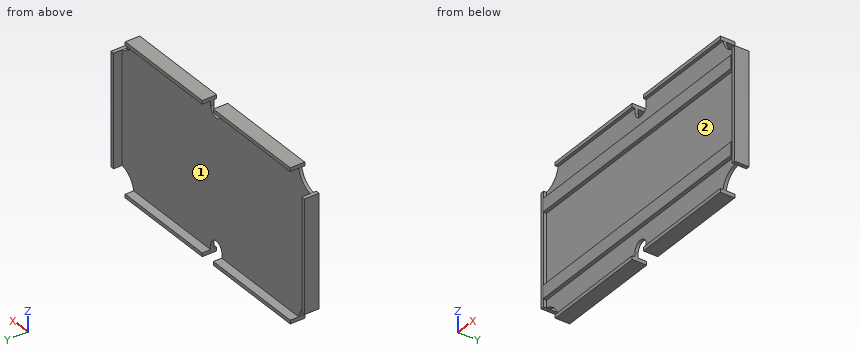
```python
from build123d import *

# Parameters (mm, degrees)
CROQUIS1_W              = 92.4
CROQUIS1_H              = 52.4
SALIENTE_EXTRUIR1_DEPTH = 5
CROQUIS2_W              = 89.9
CROQUIS2_H              = 49.9
CORTAR_EXTRUIR1_DEPTH   = 2.93
CORTAR_EXTRUIR2_START   = -2.07
CORTAR_EXTRUIR2_DEPTH   = 5
CORTAR_EXTRUIR3_START   = -2.07
CORTAR_EXTRUIR3_DEPTH   = 5
SIMETR_A2_START         = -2.07
SIMETR_A2_COPY_1_DEPTH  = 5
CORTAR_EXTRUIR5_DEPTH   = 1
CROQUIS7_W              = 89.9
CROQUIS7_H              = 4.51
SALIENTE_EXTRUIR2_DEPTH = 1.24


with BuildPart() as part:
    # Croquis1 → Saliente-Extruir1 (new body)
    with BuildSketch(Plane(origin=(0, 0, 0), x_dir=(1, 0, 0), z_dir=(0, 1, 0))):
        Rectangle(CROQUIS1_W, CROQUIS1_H)
    extrude(amount=SALIENTE_EXTRUIR1_DEPTH)

    # Croquis2 → Cortar-Extruir1 (cut)
    with BuildSketch(Plane(origin=(0, 5, 0), x_dir=(1, 0, 0), z_dir=(0, 1, 0))):
        Rectangle(CROQUIS2_W, CROQUIS2_H)
    extrude(amount=-CORTAR_EXTRUIR1_DEPTH, mode=Mode.SUBTRACT)

    # Croquis3 → Cortar-Extruir2 (cut)
    with BuildSketch(Plane(origin=(0, 2.07, 0), x_dir=(1, 0, 0), z_dir=(0, 1, 0)).offset(CORTAR_EXTRUIR2_START)):
        with BuildLine():
            Line((2.65, -23.31), (2.65, -26.2))
            Line((2.65, -26.2), (-2.65, -26.2))
            Line((-2.65, -26.2), (-2.65, -23.31))
            ThreePointArc((-2.65, -23.31), (0, -20.66), (2.65, -23.31))
        make_face()
    cortar_extruir2 = extrude(amount=CORTAR_EXTRUIR2_DEPTH, mode=Mode.SUBTRACT)

    # Croquis4 → Cortar-Extruir3 (cut)
    with BuildSketch(Plane(origin=(0, 2.07, 0), x_dir=(1, 0, 0), z_dir=(0, 1, 0)).offset(CORTAR_EXTRUIR3_START)):
        with BuildLine():
            Line((-46.2, -19.414169174), (-46.2, -26.2))
            Line((-46.2, -26.2), (-39.414169174, -26.2))
            Line((-39.414169174, -26.2), (-39.414169174, -24.95))
            ThreePointArc((-39.414169174, -24.95), (-41.32096321, -21.32096321), (-44.95, -19.414169174))
            Line((-44.95, -19.414169174), (-46.2, -19.414169174))
        make_face()
    cortar_extruir3 = extrude(amount=CORTAR_EXTRUIR3_DEPTH, mode=Mode.SUBTRACT)

    # Simetría1: Cortar-Extruir3 across plane
    add(cortar_extruir3.mirror(Plane(origin=(0, 0, 0), x_dir=(0, 0, 1), z_dir=(1, 0, 0))), mode=Mode.SUBTRACT)

    # Simetría2: Cortar-Extruir3 across plane
    add(cortar_extruir3.mirror(Plane.XY), mode=Mode.SUBTRACT)

    # Simetría2 copy 1 sketch → Simetría2 copy 1 (cut)
    with BuildSketch(Plane(origin=(0, 2.07, 0), x_dir=(-1, 0, 0), z_dir=(0, 1, 0)).offset(SIMETR_A2_START)):
        with BuildLine():
            Line((-46.2, -19.414169174), (-46.2, -26.2))
            Line((-46.2, -26.2), (-39.414169174, -26.2))
            Line((-39.414169174, -26.2), (-39.414169174, -24.95))
            ThreePointArc((-39.414169174, -24.95), (-41.32096321, -21.32096321), (-44.95, -19.414169174))
            Line((-44.95, -19.414169174), (-46.2, -19.414169174))
        make_face()
    extrude(amount=SIMETR_A2_COPY_1_DEPTH, mode=Mode.SUBTRACT)

    # Simetría3: Cortar-Extruir2 across plane
    add(cortar_extruir2.mirror(Plane.XY), mode=Mode.SUBTRACT)

    # Croquis6 → Cortar-Extruir5 (cut)
    with BuildSketch(Plane.XZ):
        with BuildLine():
            Line((2.65, -24.95), (3.9, -24.95))
            Line((3.9, -24.95), (38.164169174, -24.95))
            Line((38.164169174, -24.95), (39.414169174, -24.95))
            ThreePointArc((39.414169174, -24.95), (41.32096321, -21.32096321), (44.95, -19.414169174))
            Line((44.95, -19.414169174), (44.95, -18.164169174))
            Line((44.95, -18.164169174), (44.95, 18.164169174))
            Line((44.95, 18.164169174), (44.95, 19.414169174))
            ThreePointArc((44.95, 19.414169174), (41.32096321, 21.32096321), (39.414169174, 24.95))
            Line((39.414169174, 24.95), (38.164169174, 24.95))
            Line((38.164169174, 24.95), (3.9, 24.95))
            Line((3.9, 24.95), (2.65, 24.95))
            Line((2.65, 24.95), (2.65, 23.31))
            ThreePointArc((2.65, 23.31), (0, 20.66), (-2.65, 23.31))
            Line((-2.65, 23.31), (-2.65, 24.95))
            Line((-2.65, 24.95), (-3.9, 24.95))
            Line((-3.9, 24.95), (-38.164169174, 24.95))
            Line((-38.164169174, 24.95), (-39.414169174, 24.95))
            ThreePointArc((-39.414169174, 24.95), (-41.32096321, 21.32096321), (-44.95, 19.414169174))
            Line((-44.95, 19.414169174), (-44.95, 18.164169174))
            Line((-44.95, 18.164169174), (-44.95, -18.164169174))
            Line((-44.95, -18.164169174), (-44.95, -19.414169174))
            ThreePointArc((-44.95, -19.414169174), (-41.32096321, -21.32096321), (-39.414169174, -24.95))
            Line((-39.414169174, -24.95), (-38.164169174, -24.95))
            Line((-38.164169174, -24.95), (-3.9, -24.95))
            Line((-3.9, -24.95), (-2.65, -24.95))
            Line((-2.65, -24.95), (-2.65, -23.31))
            ThreePointArc((-2.65, -23.31), (0, -20.66), (2.65, -23.31))
            Line((2.65, -23.31), (2.65, -24.95))
        make_face()
    extrude(amount=-CORTAR_EXTRUIR5_DEPTH, mode=Mode.SUBTRACT)

    # Croquis7 → Saliente-Extruir2 (add)
    with BuildSketch(Plane.XZ.offset(-1)):
        with Locations((0, -14.565)):
            Rectangle(CROQUIS7_W, CROQUIS7_H)
    saliente_extruir2 = extrude(amount=SALIENTE_EXTRUIR2_DEPTH)

    # Simetría4: Saliente-Extruir2 across plane
    add(saliente_extruir2.mirror(Plane.XY))


solid = part.part
```
Work out the finished part from the listing and answer in its coordinate system (mm). Face numbers are marked on the shaded views. A direction names the side the tool comes from. Coordinates: 2 decimals unless noted, no trailing zeros. Write each loop counter-clockwise with the first axis right and the second up, starting at its lowest first coordinate (ties: lowest second). Pieces come first, ordered by that corner, then holes.
Q1. Which of the six approach directions +Z, -Z, +X, -X, +Y, -Y give full straight-line access (tool end or side, diameter ignored) to the marked faces 1 and 2?
Q2. Each of these flat-tipped pins is pushed along its axis until it touches: pin 1 Ø1 at (x, y) = (0, 1) entering from +Z; pin 2 Ø3 at (y, z) = (3.5, -25.5) entering from +X; pin 3 Ø0.6 at (x, y) = (45.5, 3.5) entering from -Z. Where does it stop, or does it pass through?
Q3. A cutting plane is placed at B-B, the plane x = -35. Give the vertices of the cut face in (y, z), then the cut area to 3 significant figures.
Q4. Find the intervals of material crossed by line 1 (Z direction, x = -8.5, y = 0.35); line 2 (X direction, y = 4.35, z = 1); line 3 (Z direction, x = -17, y = 4.55), in increasing order.
Q5. A cutting plane is placed at A-A, the plane z = -14. Give the vertices of the cut face in (x, y), then the cut area to 3 significant figures.
Q6. A cutting plane is placed at C-C, the plane x = 0. Give the vertices of the cut face in (y, z), then the cut area to 3 significant figures.
Findings below:
1. face 1: +Y
1. face 2: -Y
2. pin 1: stops at z = 20.71
2. pin 2: stops at x = 39.41
2. pin 3: stops at z = -19.41
3. outline: (-0.24, -16.82) - (1, -16.82) - (1, -24.95) - (0, -24.95) - (0, -26.2) - (5, -26.2) - (5, -24.95) - (2.07, -24.95) - (2.07, 24.95) - (5, 24.95) - (5, 26.2) - (0, 26.2) - (0, 24.95) - (1, 24.95) - (1, 16.82) - (-0.24, 16.82) - (-0.24, 12.31) - (1, 12.31) - (1, -12.31) - (-0.24, -12.31) - close
3. area: 77.1 mm2
4. line 1: z = -26.2 to -24.95, -16.82 to -12.31, 12.31 to 16.82, 24.95 to 26.2
4. line 2: x = -46.2 to -44.95, 44.95 to 46.2
4. line 3: z = -26.2 to -24.95, 24.95 to 26.2
5. outline: (-46.2, 0) - (-44.95, 0) - (-44.95, -0.24) - (44.95, -0.24) - (44.95, 0) - (46.2, 0) - (46.2, 5) - (44.95, 5) - (44.95, 2.07) - (-44.95, 2.07) - (-44.95, 5) - (-46.2, 5) - close
5. area: 220 mm2
6. outline: (-0.24, -16.82) - (1, -16.82) - (1, -20.66) - (2.07, -20.66) - (2.07, 20.66) - (1, 20.66) - (1, 16.82) - (-0.24, 16.82) - (-0.24, 12.31) - (1, 12.31) - (1, -12.31) - (-0.24, -12.31) - close
6. area: 55.4 mm2
